```python
from build123d import *

# Parameters (mm, degrees)
F0_R     = 1.25
F1_DEPTH = 10
F2_R     = 5.45
F2_R_2   = 1.25
F3_DEPTH = 10
F4_R     = 1.5875
F5_DEPTH = 15
F6_R     = 1.5
F7_DEPTH = 12.5


with BuildPart() as f1:
    # F0 (on Top) → F1 (new body)
    with BuildSketch(Plane.XY):
        Polygon((2.2317760525, -3.1025133052), (5.6817760525, -1.1106548765), (5.6817760525, 2.8730619809), (2.2317760525, 4.8649204096), (-1.2182239475, 2.8730619809), (-1.2182239475, -1.1106548765), align=None)
        with Locations((2.2317760525, 0.8812035522)):
            Circle(F0_R, mode=Mode.SUBTRACT)
    extrude(amount=F1_DEPTH)

    # F2 (on face) → F3 (join)
    with BuildSketch(Plane.XY.offset(10)):
        with Locations((2.2317760525, 0.8812035522)):
            Circle(F2_R)
        Polygon((2.2317760525, -3.1025133052), (-1.2182239475, -1.1106548765), (-1.2182239475, 2.8730619809), (2.2317760525, 4.8649204096), (5.6817760525, 2.8730619809), (5.6817760525, -1.1106548765), align=None, mode=Mode.SUBTRACT)
        Polygon((-1.2182239475, 2.8730619809), (-1.2182239475, -1.1106548765), (2.2317760525, -3.1025133052), (5.6817760525, -1.1106548765), (5.6817760525, 2.8730619809), (2.2317760525, 4.8649204096), align=None)
        with Locations((2.2317760525, 0.8812035522)):
            Circle(F2_R_2, mode=Mode.SUBTRACT)
        with Locations((2.2317760525, 0.8812035522)):
            Circle(F2_R_2)
    extrude(amount=F3_DEPTH)

    # F4 (on face) → F5 (cut)
    with BuildSketch(Plane.XY.offset(20)):
        with Locations((2.2317760525, 0.8812035522)):
            Circle(F4_R)
    extrude(amount=-F5_DEPTH, mode=Mode.SUBTRACT)

    # F6 (on face) → F7 (cut, symmetric)
    with BuildSketch(Plane.YZ.offset(5.6817760525)):
        with Locations((0.8812035522, 15.5740641057)):
            Circle(F6_R)
    extrude(amount=F7_DEPTH, both=True, mode=Mode.SUBTRACT)


solid = f1.part
```
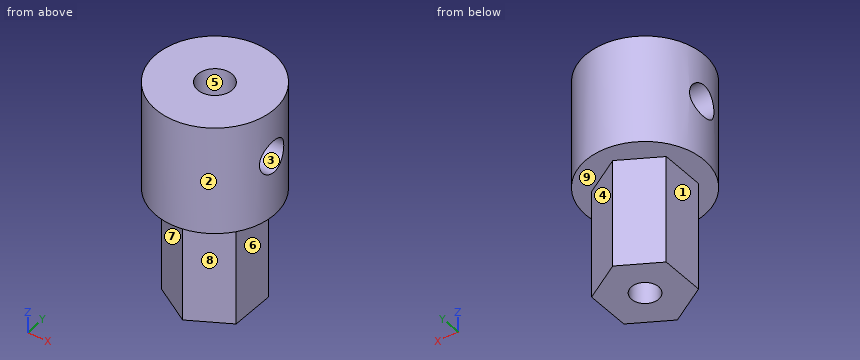
Geometry check sheet. Reference: the model listing, model coordinates, mm. Face numbers are marked on the shaded views. A direction names the side the tool comes from. Give positions to 0.01 mm unless a question says otherwise; leave off trailing zeros. Write each loop counter-clockwise with the first axis right and the second up, starting at its lowest first coordinate (ties: lowest second). Pieces come first, ordered by that corner, then holes. Notation, with made-up numbers: (23, 9.5) -> (49, 9.5) arc R24 ccw to (49, 38.5) -> close; hole circle Ø10 at (-28, 40.5). An arc over 180 degrees is marked (long way). Use one line per item in the form item = value.
Item 1: Scan lines: line 1 (Z direction, x = -2.25, y = 1); line 2 (Z direction, x = 5.75, y = -2.75); line 3 (X direction, y = -0.75, z = 7.5). Record each from-to range of solid material in increasing order.
Results list:
line_1 = 10 to 14.08, 17.07 to 20
line_2 = 10 to 20
line_3 = -1.22 to 5.68
Item 2: Sectioned sample at A-A on y = 1.75. Enter the section's corners in (x, z), plus the area to 3 significant figures.
Results list:
outline = (-3.15, 10) -> (-1.22, 10) -> (-1.22, 0) -> (1.33, 0) -> (1.33, 5) -> (0.9, 5) -> (0.9, 14.35) -> (-3.15, 14.35) -> close; (-3.15, 16.8) -> (0.9, 16.8) -> (0.9, 20) -> (-3.15, 20) -> close; (3.13, 0) -> (5.68, 0) -> (5.68, 10) -> (7.61, 10) -> (7.61, 14.35) -> (3.56, 14.35) -> (3.56, 5) -> (3.13, 5) -> close; (3.56, 16.8) -> (7.61, 16.8) -> (7.61, 20) -> (3.56, 20) -> close
area = 108 mm2
Item 3: Sectioned sample at D-D on z = 3.5. Enter the section's corners in (x, y), plus the area to 3 significant figures.
Results list:
outline = (-1.22, -1.11) -> (2.23, -3.1) -> (5.68, -1.11) -> (5.68, 2.87) -> (2.23, 4.86) -> (-1.22, 2.87) -> close; hole circle Ø2.5 at (2.23, 0.88)
area = 36.3 mm2
Item 4: Mould release check, pull along Y, two halves, no side actions. Record for the marked faces 1, 2, 3 and 4: released by +Y, released by -Y, zero draft, split by the parting line, or undercut.
Results list:
face_1 = zero draft
face_2 = split by the parting line
face_3 = undercut
face_4 = released by +Y
Item 5: Access from +Z, -Z, +X, -X, +Y, -Y to the whole of each face (thin tool, end or side, straight path). Record for the marked faces 5, 6, 7, 8 and 9.
Results list:
face_5 = +Z
face_6 = -Z, +X, +Y, -Y
face_7 = -Z, -X, -Y
face_8 = -Z, +X, -Y
face_9 = -Z
Item 6: Depth check by flat-ended pin: pin 1 Ø4.5 at (y, z) = (1.5, 7) entering from -X; pin 2 Ø2 at (x, z) = (6, 3.5) entering from -Y; pin 3 Ø3 at (y, z) = (2, 6) entering from +X; pin 4 Ø2 at (x, y) = (2.23, 0.88) entering from -Z. Enter the tip coordinate at first touch or a pass-through.
Results list:
pin_1 = -1.22
pin_2 = -1.5
pin_3 = 5.68
pin_4 = through
Item 7: Sectioned sample at C-C on x = 5. Enter the section's corners in (y, z), plus the area to 3 significant figures.
Results list:
outline = (-3.81, 10) -> (-1.5, 10) -> (-1.5, 0) -> (3.27, 0) -> (3.27, 10) -> (5.58, 10) -> (5.58, 20) -> (-3.81, 20) -> close; hole circle Ø3 at (0.88, 15.57)
area = 135 mm2
